Work out the finished part from the listing and answer in its coordinate system (mm). A direction names the side the tool comes from. Give positions to 0.01 mm unless a question says otherwise; leave off trailing zeros. Write each loop counter-clockwise with the first axis right and the second up, starting at its lowest first coordinate (ties: lowest second). Pieces come first, ordered by that corner, then holes.
1) Straight lines are drawn through the part: probe 1 along Y at (x, z) = (50.5, 7.75); probe 2 along Z at (x, y) = (-7.5, 5). For each, find the intervals that lie inside material, in ascending order.
2) A tool of negligible diameter and unlimited length cuts with its end or side. For faces 4 (the face through (-3, 72.024, 4)), 5 (the face through (-3, -24.476, 6)), from which of +Z, -Z, +X, -X, +Y, -Y can it reach the whole face along a straight path? Write none if from no direction.
3) Find section B-B (x = -56). Determine the outline of the cut face in (y, z), plus the area to 3 significant figures.
4) Determine the mould class of faces 1 (the face through (-3, -29.376, 4)), 2 (the face through (-3, 22, 0)), 3 (the face through (-3, 67.124, 6)) for opening direction Y: pulls with the +Y half, pulls with the -Y half, needs draft (parallel to the pull), parting line crosses it, or undercut.
5) Find section A-A (z = 7). Determine the outline of the cut face in (x, y), plus the area to 3 significant figures.
6) Given pin 1 Ø4 at (x, y) = (-44.5, 32.5) entering from +Z; pin 2 Ø1.2 at (x, y) = (58.31, 69.82) entering from +Z, each flat-ended and moving along its own axis, determine where each tip first touches the part or whether it passes through.
7) Find section C-C (y = 62.5). Determine the outline of the cut face in (x, z), plus the area to 4 significant figures.
```python
from build123d import *

# Parameters (mm, degrees)
F0_W     = 135.5
F0_H     = 101.4
F1_DEPTH = 3
F2_W     = 135.5
F2_H     = 4.9
F3_DEPTH = 6
F4_DEPTH = 6
F6_D     = 2
F6_DEPTH = 5
F6_TIP   = 0.600860619


with BuildPart() as f1:
    # F0 (on Top) → F1 (new body)
    with BuildSketch(Plane.XY):
        with Locations((-1.68951042, 21.3235962429)):
            Rectangle(F0_W, F0_H)
    extrude(amount=F1_DEPTH)

    # F2 (on face) → F3 (join)
    with BuildSketch(Plane.XY.offset(3)):
        with Locations((-1.68951042, -26.9264037571)):
            Rectangle(F2_W, F2_H)
    extrude(amount=F3_DEPTH)

    # F2 (on face) → F4 (join)
    with BuildSketch(Plane.XY.offset(3)):
        with Locations((-1.68951042, -26.9264037571)):
            Rectangle(F2_W, F2_H)
        with Locations((-1.68951042, 69.5735962429)):
            Rectangle(F2_W, F2_H)
    extrude(amount=F4_DEPTH)

    # F6
    with Locations(Plane.XY.offset(9)):
        with Locations((-61.68951042, 69.8235962429), (-1.68951042, 69.8235962429), (58.31048958, 69.8235962429), (58.31048958, -27.1764037571), (-1.68951042, -27.1764037571), (-61.68951042, -27.1764037571)):
            Hole(F6_D / 2, depth=F6_DEPTH)
            with Locations((0, 0, -(F6_DEPTH + F6_TIP / 2))):  # 118° drill point
                Cone(0, F6_D / 2, F6_TIP, mode=Mode.SUBTRACT)


solid = f1.part
```
Results:
1. probe 1: y = -29.38 to -24.48, 67.12 to 72.02
1. probe 2: z = 0 to 3
2. face 4: +Z, -Z, +X, -X, +Y
2. face 5: +Z, +X, -X
3. outline: (-29.38, 0) - (72.02, 0) - (72.02, 9) - (67.12, 9) - (67.12, 3) - (-24.48, 3) - (-24.48, 9) - (-29.38, 9) - close
3. area: 363 mm2
4. face 1: pulls with the -Y half
4. face 2: needs draft
4. face 3: undercut
5. outline: (-69.44, -29.38) - (66.06, -29.38) - (66.06, -24.48) - (-69.44, -24.48) - close; (-69.44, 67.12) - (66.06, 67.12) - (66.06, 72.02) - (-69.44, 72.02) - close; hole circle Ø2 at (-61.69, -27.18); hole circle Ø2 at (-61.69, 69.82); hole circle Ø2 at (-1.69, -27.18); hole circle Ø2 at (-1.69, 69.82); hole circle Ø2 at (58.31, -27.18); hole circle Ø2 at (58.31, 69.82)
5. area: 1,310 mm2
6. pin 1: stops at z = 3
6. pin 2: stops at z = 3.76
7. outline: (-69.44, 0) - (66.06, 0) - (66.06, 3) - (-69.44, 3) - close
7. area: 406.5 mm2
